```python
from build123d import *

# Parameters (mm, degrees)
SKETCH1_R               = 1.25
SKETCH1_R_2             = 2.25
BOSS_EXTRUDE1_DEPTH     = 6
CUT_EXTRUDE1_DEPTH      = 28.49545417
CUT_EXTRUDE1_DEPTH_BACK = 28.49545417
SKETCH2_W               = 8
SKETCH2_H               = 4


with BuildPart() as part:
    # Sketch1 → Boss-Extrude1 (new body)
    with BuildSketch(Plane(origin=(0, 0, 0), x_dir=(1, 0, 0), z_dir=(0, 1, 0))):
        with BuildLine():
            Line((-7, 12), (7, 12))
            ThreePointArc((7, 12), (10.535533906, 10.535533906), (12, 7))
            Line((12, 7), (12, -7))
            ThreePointArc((12, -7), (10.535533906, -10.535533906), (7, -12))
            Line((7, -12), (-7, -12))
            ThreePointArc((-7, -12), (-10.535533906, -10.535533906), (-12, -7))
            Line((-12, -7), (-12, 7))
            ThreePointArc((-12, 7), (-10.535533906, 10.535533906), (-7, 12))
        make_face()
        with Locations(Location((-5.5, 5.5, 0), (0, 0, 270))):
            Circle(SKETCH1_R, mode=Mode.SUBTRACT)
        with Locations(Location((5.5, 5.5, 0), (0, 0, 270))):
            Circle(SKETCH1_R, mode=Mode.SUBTRACT)
        with Locations(Location((5.5, -5.5, 0), (0, 0, 270))):
            Circle(SKETCH1_R, mode=Mode.SUBTRACT)
        with Locations(Location((-5.5, -5.5, 0), (0, 0, 270))):
            Circle(SKETCH1_R, mode=Mode.SUBTRACT)
        with Locations(Location((0, 0, 0), (0, 0, 270))):
            Circle(SKETCH1_R_2, mode=Mode.SUBTRACT)
    extrude(amount=BOSS_EXTRUDE1_DEPTH)

    # Sketch2 → Cut-Extrude1 (cut, two sides: drawn at the far end of the back side and taken through both)
    with BuildSketch(Plane.XY.offset(12).offset(-CUT_EXTRUDE1_DEPTH_BACK)):
        with Locations((0, 2)):
            Rectangle(SKETCH2_W, SKETCH2_H)
    extrude(amount=CUT_EXTRUDE1_DEPTH + CUT_EXTRUDE1_DEPTH_BACK, mode=Mode.SUBTRACT)


solid = part.part
```
Geometry: final body of the model. Coordinates: model frame, mm. A direction names the side the tool comes from. Give positions to 0.01 mm unless a question says otherwise; leave off trailing zeros. Write each loop counter-clockwise with the first axis right and the second up, starting at its lowest first coordinate (ties: lowest second). Pieces come first, ordered by that corner, then holes.
1. Section query D-D, the plane z = 5.5. Return loops of the section in (x, y), then the cut area to 3 significant figures.
2. Pin query (flat end, axial travel): P1, Ø2, axis at y = 3.5, z = -8.5, coming from the -X side; P2, Ø2, axis at x = -5.5, z = -5.5, coming from the -Y side; P3, Ø2, axis at x = 0.5, z = 3, coming from the -Y side. Return the tip coordinate at first contact, or that it passes through.
3. Reachability of faces 4 (the flat face through (-8, 0, 0)), 5 (the flat face through (0, 4, -3)) from +Z, -Z, +X, -X, +Y, -Y: full face, straight path, thin tool, end or side. Return the list, or none.
4. Section query C-C, the plane x = 5.5. Return loops of the section in (y, z), then the cut area to 3 significant figures.
5. Draft query along X for faces 1 (the cylindrical face through (4.28, 2.96, -5.77)), 2 (the flat face through (-2.5, 6, -0.2)), 3 (the flat face through (-12, 3, 0)). Return one class per face: released by +X, released by -X, zero draft, split by the parting line, or undercut.
6. Section query A-A, the plane y = 3.5. Return loops of the section in (x, z).
7. Line query: probe 1 along X at (y, z) = (4.85, 5.5); probe 2 along X at (y, z) = (1.45, -5.5); probe 3 along X at (y, z) = (5.4, 0). Output: solid intervals per line, ascending.
8. Section query B-B, the plane z = 0. Return loops of the section in (x, y), then the cut area to 3 significant figures.
Computed:
1. outline: (-12, 0) - (-6.75, 0) - (-6.75, 6) - (-12, 6) - close; (-4.25, 0) - (-4, 0) - (-4, 4) - (4, 4) - (4, 0) - (4.25, 0) - (4.25, 6) - (-4.25, 6) - close; (6.75, 0) - (12, 0) - (12, 6) - (6.75, 6) - close
1. area: 82.0 mm2
2. P1: stops at x = -11.97
2. P2: passes through
2. P3: stops at y = 4
3. face 4: +Z, -Z, +X, -X, -Y
3. face 5: +Z, -Z, -Y
4. outline: (0, -12) - (6, -12) - (6, -6.75) - (0, -6.75) - close; (0, -4.25) - (6, -4.25) - (6, 4.25) - (0, 4.25) - close; (0, 6.75) - (6, 6.75) - (6, 12) - (0, 12) - close
4. area: 114 mm2
5. face 1: undercut
5. face 2: zero draft
5. face 3: released by -X
6. outline: (-12, -7) arc R5 ccw to (-7, -12) - (-4, -12) - (-4, 12) - (-7, 12) arc R5 ccw to (-12, 7) - close; (4, -12) - (7, -12) arc R5 ccw to (12, -7) - (12, 7) arc R5 ccw to (7, 12) - (4, 12) - close; hole circle Ø2.5 at (-5.5, -5.5); hole circle Ø2.5 at (-5.5, 5.5); hole circle Ø2.5 at (5.5, -5.5); hole circle Ø2.5 at (5.5, 5.5)
7. probe 1: x = -12 to -6.75, -4.25 to 4.25, 6.75 to 12
7. probe 2: x = -12 to -6.75, -4.25 to -4, 4 to 4.25, 6.75 to 12
7. probe 3: x = -12 to -2.25, 2.25 to 12
8. outline: (-12, 0) - (-4, 0) - (-4, 4) - (-2.25, 4) - (-2.25, 6) - (-12, 6) - close; (2.25, 4) - (4, 4) - (4, 0) - (12, 0) - (12, 6) - (2.25, 6) - close
8. area: 103 mm2
